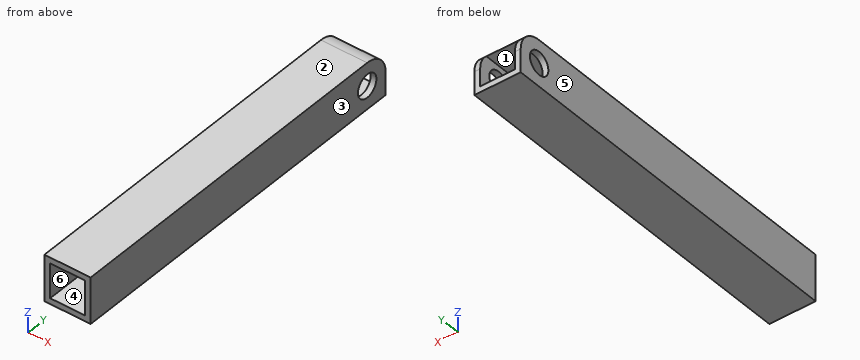
```python
from build123d import *

# Parameters (mm, degrees)
SKETCH1_W           = 25.4
SKETCH1_H           = 25.4
SKETCH1_W_2         = 19.05
SKETCH1_H_2         = 19.05
EXTRUDE_THIN1_DEPTH = 203.2
SKETCH2_R           = 6.35
CUT_EXTRUDE1_DEPTH  = 206.174779152
CUT_EXTRUDE3_DEPTH  = 206.174779152


with BuildPart() as part:
    # Sketch1 → Extrude-Thin1 (new body)
    with BuildSketch(Plane(origin=(0, 0, 0), x_dir=(1, 0, 0), z_dir=(0, 1, 0))):
        Rectangle(SKETCH1_W, SKETCH1_H)
        Rectangle(SKETCH1_W_2, SKETCH1_H_2, mode=Mode.SUBTRACT)
    extrude(amount=EXTRUDE_THIN1_DEPTH)

    # Sketch2 → Cut-Extrude1 (cut, through all)
    with BuildSketch(Plane(origin=(12.7, 0, 0), x_dir=(0, 0, -1), z_dir=(1, 0, 0))):
        with Locations((0, 190.5)):
            Circle(SKETCH2_R)
    extrude(amount=-CUT_EXTRUDE1_DEPTH, mode=Mode.SUBTRACT)

    # Sketch4 → Cut-Extrude3 (cut, through all)
    with BuildSketch(Plane(origin=(12.7, 0, 0), x_dir=(0, 0, -1), z_dir=(1, 0, 0))):
        with BuildLine():
            Line((-12.7, 190.5), (-12.7, 203.2))
            Line((-12.7, 203.2), (0, 203.2))
            ThreePointArc((0, 203.2), (-8.980256121, 199.480256121), (-12.7, 190.5))
        make_face()
    extrude(amount=-CUT_EXTRUDE3_DEPTH, mode=Mode.SUBTRACT)


solid = part.part
```
Design review of the part built by this model. Coordinates are the model's own, in mm. Face numbers are marked on the shaded views. A direction names the side the tool comes from. Coordinates: 2 decimals unless noted, no trailing zeros. Loops run counter-clockwise (first coordinate to the right, second up) from the corner with the lowest first, then second, coordinate; pieces in that order, holes last.
Q1. We need section B-B on y = 115.5. State the section outline as (x, z) points (3 decimals).
Reported:
outline: (-12.7, -12.7) - (12.7, -12.7) - (12.7, 12.7) - (-12.7, 12.7) - close; hole (-9.525, -9.525) - (9.525, -9.525) - (9.525, 9.525) - (-9.525, 9.525) - close
Q2. Tool access review of the marked faces 5 and 6: name each direction out of +Z, -Z, +X, -X, +Y, -Y from which nothing blocks a thin tool from reaching the whole face with its end or side.
Reported:
face 5: +Z, -Z, -X, +Y, -Y
face 6: +Y, -Y
Q3. We need section A-A on x = -7. State the section outline as (y, z) points (3 decimals).
Reported:
outline: (0, -12.7) - (203.2, -12.7) - (203.2, -9.525) - (0, -9.525) - close; (0, 9.525) - (198.9, 9.525) arc R12.7 ccw to (190.5, 12.7) - (0, 12.7) - close
Q4. For pin 1 (10 mm diameter, centred on x = 3.5, z = -9.5, fed in from +Y); pin 2 (11.5 mm diameter, centred on y = 190.5, z = 0, fed in from +X), all flat-tipped, find the tip position at first contact; note any pin that passes through.
Reported:
pin 1: stops at y = 203.2
pin 2: passes through
Q5. The part is to be moulded in two halves that separate along Z. For the marked faces 1, 2, 3 and 4, say which applies: +Z half, -Z half, draft (parallel to the pull), parting line (faces both ways), or undercut.
Reported:
face 1: undercut
face 2: +Z half
face 3: draft
face 4: undercut
Q6. We need section C-C on z = 3.5. State the section outline as (x, y) points (3 decimals).
Reported:
outline: (-12.7, 0) - (-9.525, 0) - (-9.525, 185.202) - (-12.7, 185.202) - close; (-12.7, 195.798) - (-9.525, 195.798) - (-9.525, 202.708) - (-12.7, 202.708) - close; (9.525, 0) - (12.7, 0) - (12.7, 185.202) - (9.525, 185.202) - close; (9.525, 195.798) - (12.7, 195.798) - (12.7, 202.708) - (9.525, 202.708) - close
Q7. To check wall thickness, follow line 1 (Z direction, x = -5.5, y = 48) (3 decimals); line 2 (Y direction, x = 10.35, z = 0). State the ranges of each line that lie inside material, in increasing order.
Reported:
line 1: z = -12.7 to -9.525, 9.525 to 12.7
line 2: y = 0 to 184.15, 196.85 to 203.2
